from build123d import *

# Parameters (mm, degrees)
SKICA1_RX               = 60
SKICA1_RY               = 30
SKICA1_R                = 4
P_IDAT_VYSUNUT_M1_DEPTH = 10
SKICA1_4_R              = 4
P_IDAT_VYSUNUT_M3_DEPTH = 10
CRVPATTERN1_START       = -10
CRVPATTERN1_OUTLINE_R   = 4
CRVPATTERN1_DEPTH       = 10


# Read off the part's stored shape, not the designer's step: CrvPattern1
with BuildPart() as part:
    # Skica1 → Přidat vysunutím1 (new body)
    # profile 1 of 2: a face of its own
    with BuildSketch(Plane.XY):
        with Locations((0, 0)):
            Ellipse(SKICA1_RX, SKICA1_RY)
        with Locations((-50, 0)):
            Circle(SKICA1_R, mode=Mode.SUBTRACT)
    # profile 2 of 2: a face of its own
    with BuildSketch(Plane.XY):
        with Locations((-50, 0)):
            Circle(SKICA1_R)
    extrude(amount=P_IDAT_VYSUNUT_M1_DEPTH)

    # Skica1<4> → Přidat vysunutím3 (add)
    with BuildSketch(Plane.XY):
        with Locations((-50, 0)):
            Circle(SKICA1_4_R)
    extrude(amount=-P_IDAT_VYSUNUT_M3_DEPTH)

    # CrvPattern1 outline → CrvPattern1 (add)
    with BuildSketch(Plane.XY.offset(CRVPATTERN1_START)):
        with Locations((-33.492839023, 14.250541881)):
            Circle(CRVPATTERN1_OUTLINE_R)
        with Locations((-11.370922058, 19.405478737)):
            Circle(CRVPATTERN1_OUTLINE_R)
        with Locations((11.370433267, 19.405524946)):
            Circle(CRVPATTERN1_OUTLINE_R)
        with Locations((33.493372943, 14.250403108)):
            Circle(CRVPATTERN1_OUTLINE_R)
        with Locations((49.999827835, -8.0151e-05)):
            Circle(CRVPATTERN1_OUTLINE_R)
        with Locations((33.493062429, -14.250407673)):
            Circle(CRVPATTERN1_OUTLINE_R)
        with Locations((11.369477866, -19.405634054)):
            Circle(CRVPATTERN1_OUTLINE_R)
        with Locations((-11.370751059, -19.405496472)):
            Circle(CRVPATTERN1_OUTLINE_R)
        with Locations((-33.492737691, -14.250555974)):
            Circle(CRVPATTERN1_OUTLINE_R)
    extrude(amount=CRVPATTERN1_DEPTH)


solid = part.part
Geometry: final body of the model. Coordinates: model frame, mm. A direction names the side the tool comes from. Round coordinates to 2 decimals unless told otherwise and drop trailing zeros.
Q1. Material intervals for L1, parallel to X at y = -19, z = -7.5; L2, parallel to Z at x = 29, y = -14; L3, parallel to X at y = 3.5, z = -1, sorted ascending.
Q2. Pin query (flat end, axial travel): P1, Ø3, axis at y = 11, z = -7.5, coming from the +X side; P2, Ø10, axis at x = -37.5, y = 5.5, coming from the -Z side; P3, Ø1.5, axis at y = 16.5, z = 1.5, coming from the -X side. Return the tip coordinate at first contact, or that it passes through.
Q3. Access query for faces 1 (the cylindrical face through (-11.89, 23.37, -5.07)), 2 (the flat face through (-34, 14, -10)). Directions: +Z, -Z, +X, -X, +Y, -Y. A direction counts if a zero-diameter tool reaches every point of the face in a straight line with its end or side. Return the directions, or none.
Q4. Pull-direction query (X, two-part tool) for faces 3 (the cylindrical face through (-14.545, -21.839, -5.07)), 4 (the flat face through (-1, 0, 10)); classes: released by +X, released by -X, zero draft, split by the parting line, or undercut.
Q5. Section A-A on z = -1.75. State how many separate pieces and enclosed holes the cut face has, plus the area to 3 significant figures.
Evaluation:
1. L1: x = -15.35 to -7.39, 7.39 to 15.35
1. L2: z = 0 to 10
1. L3: x = -51.94 to -48.06, 48.06 to 51.94
2. P1: stops at x = 37.09
2. P2: stops at z = 0
2. P3: stops at x = -51.07
3. face 1: -Z
3. face 2: -Z, +X, -X, +Y, -Y
4. face 3: undercut
4. face 4: zero draft
5. separate pieces: 10
5. enclosed holes: 0
5. area: 503 mm2
